Input: part model. Units: mm. Frame: model coordinates. Face numbers are marked on the shaded views. A direction names the side the tool comes from. Coordinates: 2 decimals unless noted, no trailing zeros. Loops run counter-clockwise (first coordinate to the right, second up) from the corner with the lowest first, then second, coordinate; pieces in that order, holes last.
(1) Section C-C, the plane y = 0.3. Return loops of the section in (x, z).
(2) Section D-D, the plane y = 1.15. Return loops of the section in (x, z).
(3) Set-up query: the marked faces 5 and 6. Return all of +Z, -Z, +X, -X, +Y, -Y with unobstructed straight access to the full face (end or side cutting, diameter ignored); none if empty.
(4) Contact query for flat-ended pins moving along their axis: P1, Ø6, axis at x = 0, z = 0, coming from the +Y side; P2, Ø1, axis at x = 1, y = 2, coming from the -Z side. Output: stop coordinate, or through.
(5) Mould query, pull axis X, two halves, no side actions, for the marked faces 1, 2, 3 and 4. Classes: released by +X, released by -X, zero draft, split by the parting line, or undercut.
(6) Line query: L1, parallel to X at y = 2.8, z = 0; L2, parallel to Y at x = -3, z = -2; L3, parallel to Y at x = -2.25, z = 4.25. Output: solid intervals per line, ascending.
```python
from build123d import *


with BuildPart() as f1:
    # F0 (on Right) → F1 (revolve)
    with BuildSketch(Plane.YZ):
        Polygon((0, 2.667), (0, 1.5), (3, 1.5), (3, 2.667), (2.5, 2.667), (2.5, 3.834), (3, 3.834), (3, 5), (2.325, 5), (1.5, 4.55), (0.675, 5), (0, 5), (0, 3.834), (0.5, 3.834), (0.5, 2.667), align=None)
    revolve(axis=Axis((0, 1.5, 0), (0, 1, 0)))


solid = f1.part
```
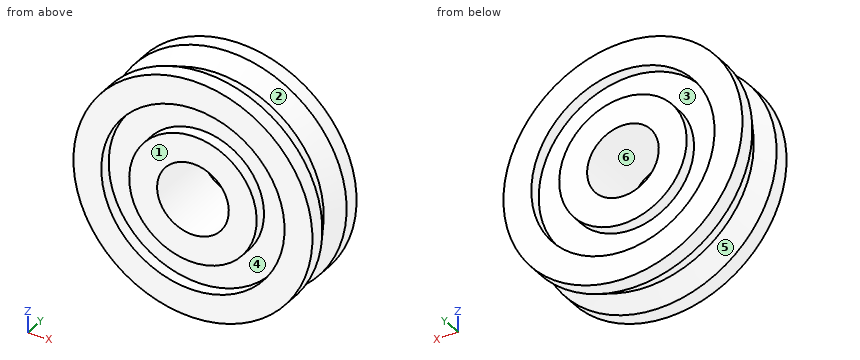
Report:
1. outline: circle Ø10 at (0, 0); circle Ø5.33 at (0, 0); hole circle Ø7.67 at (0, 0); hole circle Ø3 at (0, 0)
2. outline: circle Ø9.48 at (0, 0); hole circle Ø3 at (0, 0)
3. face 5: none
3. face 6: +Y, -Y
4. P1: stops at y = 3
4. P2: stops at z = -4.96
5. face 1: zero draft
5. face 2: split by the parting line
5. face 3: undercut
5. face 4: undercut
6. L1: x = -5 to -3.83, -2.67 to -1.5, 1.5 to 2.67, 3.83 to 5
6. L2: y = 0.5 to 2.5
6. L3: y = 0 to 1.03, 1.97 to 3
